Work out the finished part from the listing and answer in its coordinate system (mm). Face numbers are marked on the shaded views. A direction names the side the tool comes from. Round coordinates to 2 decimals unless told otherwise and drop trailing zeros. Order: outer loops, then holes, each group sorted by start corner. A loop starts at its lowest first (then second) coordinate and runs counter-clockwise, first axis right, second up. Notation, with made-up numbers: M 46.5,51.5 L 64.5,51.5 A19 ccw 64.5,88.5 Z; hole C 44,53.5 d1. An arc over 180 degrees is marked long. Return JSON: item names as keys, results as strings.
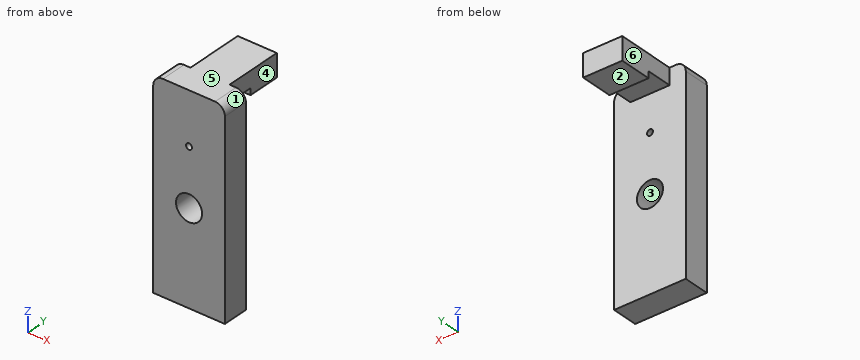
from build123d import *

# Parameters (mm, degrees)
F0_R     = 4
F1_DEPTH = 8
F2_DEPTH = 16
F3_START = -16
F3_DEPTH = 10


with BuildPart() as f1:
    # F0 (on Front) → F1 (new body)
    with BuildSketch(Plane.XZ):
        with BuildLine():
            Line((11, -17.5), (11, 17.5))
            Line((11, 17.5), (11, 30.5))
            ThreePointArc((11, 30.5), (10.1213203436, 32.6213203436), (8, 33.5))
            Line((8, 33.5), (6, 33.5))
            Line((6, 33.5), (6, 28.5))
            Line((6, 28.5), (6, 26.5))
            Line((6, 26.5), (-6, 26.5))
            Line((-6, 26.5), (-6, 28.5))
            Line((-6, 28.5), (-6, 33.5))
            Line((-6, 33.5), (-8, 33.5))
            ThreePointArc((-8, 33.5), (-10.1213203436, 32.6213203436), (-11, 30.5))
            Line((-11, 30.5), (-11, 28.5))
            Line((-11, 28.5), (-11, 17.5))
            Line((-11, 17.5), (-11, -17.5))
            Line((-11, -17.5), (-11, -28.5))
            Line((-11, -28.5), (0, -28.5))
            Line((0, -28.5), (11, -28.5))
            Line((11, -28.5), (11, -17.5))
        make_face()
        Circle(F0_R, mode=Mode.SUBTRACT)
        with BuildLine():
            ThreePointArc((0, 18.4210526316), (0.6512825616, 18.1512825616), (0.9210526316, 17.5))
            ThreePointArc((0.9210526316, 17.5), (-0.6512825616, 16.8487174384), (0, 18.4210526316))
        make_face(mode=Mode.SUBTRACT)
        Polygon((6, 26.5), (6, 28.5), (0, 28.5), (-6, 28.5), (-6, 26.5), align=None)
        Polygon((6, 28.5), (6, 33.5), (0, 33.5), (-6, 33.5), (-6, 28.5), (0, 28.5), align=None)
    extrude(amount=-F1_DEPTH)

    # F0 (on Front) → F2 (join)
    with BuildSketch(Plane.XZ):
        Polygon((6, 28.5), (6, 33.5), (0, 33.5), (-6, 33.5), (-6, 28.5), (0, 28.5), align=None)
    extrude(amount=-F2_DEPTH)

    # F0 (on Front) → F3 (join)
    with BuildSketch(Plane.XZ.offset(F3_START)):
        Polygon((6, 28.5), (6, 33.5), (0, 33.5), (-6, 33.5), (-6, 28.5), (0, 28.5), align=None)
        Polygon((6, 26.5), (6, 28.5), (0, 28.5), (-6, 28.5), (-6, 26.5), align=None)
    extrude(amount=-F3_DEPTH)


solid = f1.part
Item 1: Find section B-B (y = 5.25). Determine the outline of the cut face in (x, z), plus the area to 3 significant figures.
Output:
{"outline": "M -11,-28.5 L 11,-28.5 L 11,30.5 A3 ccw 8,33.5 L -8,33.5 A3 ccw -11,30.5 Z; hole C 0,0 d8; hole C 0,17.5 d1.84", "area": "1,310 mm^2"}
Item 2: Find section C-C (x = -1.5). Determine the outline of the cut face in (y, z).
Output:
{"outline": "M 0,-28.5 L 8,-28.5 L 8,-3.71 L 0,-3.71 Z; M 0,3.71 L 8,3.71 L 8,28.5 L 16,28.5 L 16,26.5 L 26,26.5 L 26,33.5 L 0,33.5 Z"}
Item 3: Which of the six approach directions +Z, -Z, +X, -X, +Y, -Y give full straight-line access (tool end or side, diameter ignored) to the marked faces 1 and 2?
Output:
{"face 1": "+Z, +X, +Y, -Y", "face 2": "-Z, +X, -X, +Y"}
Item 4: Find section D-D (y = 22.5). Determine the outline of the cut face in (x, z).
Output:
{"outline": "M -6,26.5 L 6,26.5 L 6,33.5 L -6,33.5 Z"}
Item 5: Each of these flat-tipped pins is pushed along its axis until it touches: pin 1 (12 mm diameter, centred on x = 1, z = -7, fed in from +Y); pin 2 (8 mm diameter, centred on x = 0.5, y = 19, fed in from -Z); pin 3 (7.5 mm diameter, centred on y = 15, z = 29.5, fed in from +X). Where does it stop, or does it pass through?
Output:
{"pin 1": "stops at y = 8", "pin 2": "stops at z = 26.5", "pin 3": "stops at x = 6"}
Item 6: Consider line 1 along Z through (x, y) = (0, 5.5); line 2 along X through (y, z) = (6.5, 17.5); line 3 along Y through (x, z) = (9.25, 15). Determine where each line is inside the solid, lowest interval first. Write a range as [from, to].
Output:
{"line 1": "z = [-28.5, -4], [4, 16.58], [18.42, 33.5]", "line 2": "x = [-11, -0.92], [0.92, 11]", "line 3": "y = [0, 8]"}
Item 7: The mould has two halves that part along X. Classify the marked faces 3, 4, 5 and 6: pulls with the +X half, pulls with the -X half, needs draft (parallel to the pull), parting line crosses it, or undercut.
Output:
{"face 3": "undercut", "face 4": "pulls with the +X half", "face 5": "needs draft", "face 6": "pulls with the -X half"}
Item 8: Find section A-A (z = 0). Determine the outline of the cut face in (x, y), plus the area to 3 significant figures.
Output:
{"outline": "M -11,0 L -4,0 L -4,8 L -11,8 Z; M 4,0 L 11,0 L 11,8 L 4,8 Z", "area": "112 mm^2"}
